```python
from build123d import *

# Parameters (mm, degrees)
SKETCH1_W               = 45.085
SKETCH1_H               = 19.05
BOSS_EXTRUDE1_DEPTH     = 10.16
SKETCH2_W               = 15
SKETCH2_H               = 15
CUT_EXTRUDE1_DEPTH      = 27.497462732
FILLET1_R               = 3.175
CUT_EXTRUDE2_DEPTH      = 27.497462732
CUT_EXTRUDE2_DEPTH_BACK = 1.016
CUT_EXTRUDE3_DEPTH      = 8.636


with BuildPart() as part:
    # Sketch1 → Boss-Extrude1 (new body)
    with BuildSketch(Plane(origin=(0, 0, 0), x_dir=(1, 0, 0), z_dir=(0, 1, 0))):
        Rectangle(SKETCH1_W, SKETCH1_H)
    extrude(amount=-BOSS_EXTRUDE1_DEPTH)

    # Sketch2 → Cut-Extrude1 (cut, through all)
    with BuildSketch(Plane(origin=(0, 0, 0), x_dir=(1, 0, 0), z_dir=(0, 1, 0))):
        Rectangle(SKETCH2_W, SKETCH2_H)
    extrude(amount=-CUT_EXTRUDE1_DEPTH, mode=Mode.SUBTRACT)

    # Fillet1
    fillet1_edges = [part.edges().sort_by_distance(p)[0] for p in [
        (22.5425, -5.08, 9.525),
        (-22.5425, -5.08, 9.525),
        (-22.5425, -5.08, -9.525),
        (22.5425, -5.08, -9.525),
    ]]
    fillet(fillet1_edges, radius=FILLET1_R)

    # Sketch3 → Cut-Extrude2 (cut, two sides: drawn at the far end of the back side and taken through both)
    with BuildSketch(Plane(origin=(0, 0, 0), x_dir=(1, 0, 0), z_dir=(0, 1, 0)).offset(-CUT_EXTRUDE2_DEPTH_BACK)):
        Polygon((-14.5425, -102.908445), (-14.5425, -9.525), (-14.5425, 9.525), (-14.5425, 102.908445), (-201.309389999, 102.908445), (-201.309389999, -102.908445), align=None)
    extrude(amount=CUT_EXTRUDE2_DEPTH + CUT_EXTRUDE2_DEPTH_BACK, mode=Mode.SUBTRACT)

    # Sketch5 → Cut-Extrude3 (cut)
    with BuildSketch(Plane.XZ.offset(10.16)):
        Polygon((-21.216, -3.666174209), (-14.866, -7.332348419), (-8.516, -3.666174209), (-8.516, 3.666174209), (-14.866, 7.332348419), (-21.216, 3.666174209), align=None)
        Polygon((8.516, -3.666174209), (14.866, -7.332348419), (21.216, -3.666174209), (21.216, 3.666174209), (14.866, 7.332348419), (8.516, 3.666174209), align=None)
    extrude(amount=-CUT_EXTRUDE3_DEPTH, mode=Mode.SUBTRACT)


solid = part.part
```
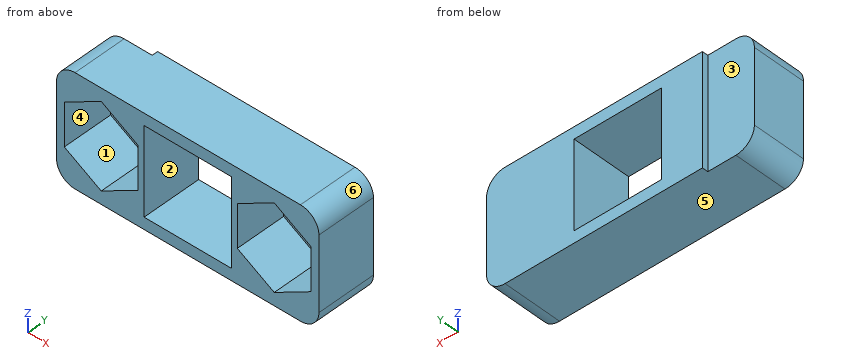
The model under review builds one solid part; all positions refer to its coordinate system, in mm. Face numbers are marked on the shaded views. A direction names the side the tool comes from. Coordinates: 2 decimals unless noted, no trailing zeros. Write each loop counter-clockwise with the first axis right and the second up, starting at its lowest first coordinate (ties: lowest second). Pieces come first, ordered by that corner, then holes.
1) Clearance check with flat-ended pins moving along their axes: pin 1 Ø0.5 at (y, z) = (-0.5, -1.5) entering from -X; pin 2 Ø6.5 at (x, z) = (14, -2.5) entering from -Y; pin 3 Ø6.5 at (x, z) = (-18.5, -4.5) entering from +Y. State where each tip first meets the part, or that it passes through.
2) We need section D-D on x = -10. State the section outline as (y, z) points (3 decimals).
3) Machinability: for the marked faces 1, 2 and 3, which of the approach directions +Z, -Z, +X, -X, +Y, -Y give a long, thin tool a straight path to every point of the face, cutting with its end or side? Answer none if there is none.
4) We need section C-C on x = -16. State the section outline as (y, z) points (3 decimals).
5) We need section B-B on y = -7.5. Count the separate pieces of the cut face and the enclosed holes in it, then the cut area to 3 significant figures.
6) To check wall thickness, follow probe 1 along X at (y, z) = (-9, 0.5); probe 2 along X at (y, z) = (-2, -5.5); probe 3 along Z at (x, y) = (-5, -8) (3 decimals). State the ranges of each line that lie inside material, in increasing order.
7) The part is to be moulded in two halves that separate along Z. For the marked faces 4, 5 and 6, say which applies: pulls with the +Z half, pulls with the -Z half, needs draft (parallel to the pull), parting line crosses it, or undercut.
8) We need section A-A on z = -1. State the section outline as (x, y) points, then the cut area to 3 significant figures.
Answer list:
1. pin 1: stops at x = -14.54
1. pin 2: stops at y = -1.52
1. pin 3: stops at y = -1.02
2. outline: (-10.16, -9.525) - (0, -9.525) - (0, 9.525) - (-10.16, 9.525) - (-10.16, 4.523) - (-1.524, 4.523) - (-1.524, -4.523) - (-10.16, -4.523) - close
3. face 1: -Y
3. face 2: +Y, -Y
3. face 3: +Z, -Z, -X, +Y
4. outline: (-10.16, -9.525) - (-1.016, -9.525) - (-1.016, 9.525) - (-10.16, 9.525) - (-10.16, 6.678) - (-1.524, 6.678) - (-1.524, -6.678) - (-10.16, -6.678) - close
5. separate pieces: 1
5. enclosed holes: 3
5. area: 346 mm2
6. probe 1: x = -22.54 to -21.22, -8.52 to -7.5, 7.5 to 8.52, 21.22 to 22.54
6. probe 2: x = -22.54 to -18.04, -11.69 to -7.5, 7.5 to 11.69, 18.04 to 22.54
6. probe 3: z = -9.525 to -7.5, 7.5 to 9.525
7. face 4: undercut
7. face 5: pulls with the -Z half
7. face 6: pulls with the +Z half
8. outline: (-22.54, -10.16) - (-21.22, -10.16) - (-21.22, -1.52) - (-8.52, -1.52) - (-8.52, -10.16) - (-7.5, -10.16) - (-7.5, 0) - (-14.54, 0) - (-14.54, -1.02) - (-22.54, -1.02) - close; (7.5, -10.16) - (8.52, -10.16) - (8.52, -1.52) - (21.22, -1.52) - (21.22, -10.16) - (22.54, -10.16) - (22.54, 0) - (7.5, 0) - close
8. area: 78.2 mm2
